Read the model definition and answer for the solid it produces. Units are mm, in the model's axes. Face numbers are marked on the shaded views. Coordinates: 2 decimals unless noted, no trailing zeros. Write each loop counter-clockwise with the first axis right and the second up, starting at its lowest first coordinate (ties: lowest second). Pieces come first, ordered by that corner, then holes. Notation, with made-up numbers: (15, 63) -> (62, 63) arc R26 ccw to (62, 85) -> close; hole circle Ø11 at (3.5, -34). An arc over 180 degrees is marked (long way). Answer in a Markdown table with one row per item. Add a question column.
Item 1: Given pin 1 Ø8 at (x, z) = (2, -8) entering from -Y; pin 2 Ø6 at (x, y) = (-2.5, 22.5) entering from -Z; pin 3 Ø2 at (x, z) = (5.5, 25) entering from +Y, each flat-ended and moving along its own axis, determine where each tip first touches the part or whether it passes through.
Item 2: For a pull along Y with two mould halves and no side action, classify the marked faces 1, 2 and 3 as +Y half, -Y half, draft (parallel to the pull), parting line (faces both ways), or undercut.
Item 3: Section D-D on y = 12 is taken. Write down the section's boundary in (x, z).
Item 4: Straight lines are drawn through the part: line 1 (Y direction, x = 0, z = 0); line 2 (Y direction, x = 2.5, z = -30.5); line 3 (Y direction, x = -2.75, z = 3). For each, find the intervals that lie inside material, in ascending order. Write a range as from..to.
Item 5: Section A-A on z = 0 is taken. Write down the section's boundary in (x, y), then the cut area to 3 significant figures.
Item 6: Section C-C on x = 0 is taken. Count the separate pieces of the cut face and the enclosed holes in it, then the cut area to 3 significant figures.
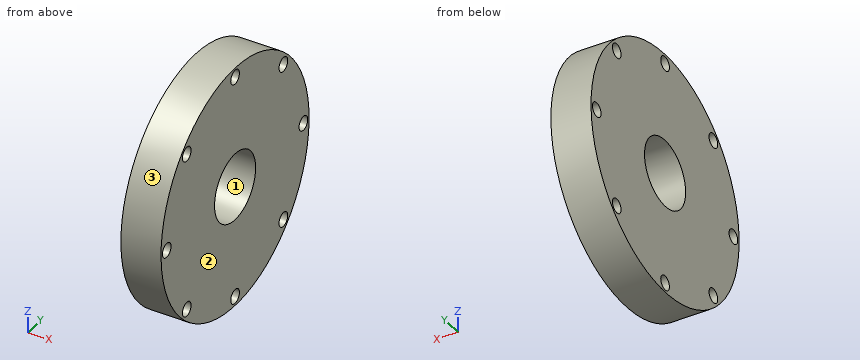
```python
from build123d import *

# Parameters (mm, degrees)
F0_W     = 15.7906897366
F0_H     = 34.8864039406
F3_R     = 2.8270891362
F4_DEPTH = 25.4
F5_COUNT = 8


with BuildPart() as f2:
    # F0 (on Front) → F2 (revolve)
    with BuildSketch(Plane.XZ):
        with Locations((-0.5508437753, 30.8469277807)):
            Rectangle(F0_W, F0_H)
    revolve(axis=Axis((-24.62522313, 0, 0), (-1, 0, 0)))

    # F3 (on face) → F4 (cut)
    with BuildSketch(Plane(origin=(-8.4461886436, 0, 0), x_dir=(0, -1, 0), z_dir=(-1, 0, 0))):
        with Locations((0, 44.5668138564)):
            Circle(F3_R)
    f4 = extrude(amount=-F4_DEPTH, mode=Mode.SUBTRACT)

    # F5: F4 ×8 about axis
    f5_axis = Axis((-8.4461886436, 0, 0), (-1, 0, 0))
    for i in range(1, F5_COUNT):
        add(f4.rotate(f5_axis, i * 360 / F5_COUNT), mode=Mode.SUBTRACT)


solid = f2.part
```
Results below:
| question | item | result |
|---|---|---|
| 1 | pin 1 | stops at y = -48.12 |
| 1 | pin 2 | stops at z = -44.18 |
| 1 | pin 3 | stops at y = 41.9 |
| 2 | face 1 | undercut |
| 2 | face 2 | draft |
| 2 | face 3 | parting line |
| 3 | outline | (-8.45, -46.78) -> (7.34, -46.78) -> (7.34, -5.97) -> (-8.45, -5.97) -> close; (-8.45, 5.97) -> (7.34, 5.97) -> (7.34, 46.78) -> (-8.45, 46.78) -> close |
| 4 | line 1 | y = -48.29..-47.39, -41.74..-13.4, 13.4..41.74, 47.39..48.29 |
| 4 | line 2 | y = -37.44..-34.15, -28.87..28.87, 34.15..37.44 |
| 4 | line 3 | y = -48.2..-13.06, 13.06..48.2 |
| 5 | outline | (-8.45, -48.29) -> (7.34, -48.29) -> (7.34, -47.39) -> (-8.45, -47.39) -> close; (-8.45, -41.74) -> (7.34, -41.74) -> (7.34, -13.4) -> (-8.45, -13.4) -> close; (-8.45, 13.4) -> (7.34, 13.4) -> (7.34, 41.74) -> (-8.45, 41.74) -> close; (-8.45, 47.39) -> (7.34, 47.39) -> (7.34, 48.29) -> (-8.45, 48.29) -> close |
| 5 | area | 923 mm2 |
| 6 | separate pieces | 1 |
| 6 | enclosed holes | 9 |
| 6 | area | 6,560 mm2 |
